from build123d import *

# Parameters (mm, degrees)
F1_DEPTH  = 12
F2_START  = 3
F2_DEPTH  = 6
F3_D      = 6.7564
F5_START  = -6
F5_DEPTH  = 4
F6_D      = 3.3
F6_DEPTH  = 8
F6_TIP    = 0.9914200214
F7_D      = 6
F7_DEPTH  = 1.5
F7_TIP    = 1.8025818571
F9_START  = -6
F9_DEPTH  = 4
F10_D     = 3.3
F10_DEPTH = 8
F10_TIP   = 0.9914200214
F11_D     = 6
F11_DEPTH = 1.5
F11_TIP   = 1.8025818571
F13_START = -6
F13_DEPTH = 4
F14_D     = 6
F14_DEPTH = 1.5
F14_TIP   = 1.8025818571
F15_D     = 3.3
F15_DEPTH = 8
F15_START = 2.3111618
F15_TIP   = 0.9914200214


with BuildPart() as f1:
    # F0 (on Front) → F1 (new body)
    with BuildSketch(Plane.XZ):
        with BuildLine():
            Line((3, -59.9289579419), (53.4, 27.3664027596))
            ThreePointArc((53.4, 27.3664027596), (51.2038475773, 29.5625551823), (50.4, 32.5625551823))
            Line((50.4, 32.5625551823), (-50.4, 32.5625551823))
            ThreePointArc((-50.4, 32.5625551823), (-51.2038475773, 29.5625551823), (-53.4, 27.3664027596))
            Line((-53.4, 27.3664027596), (-3, -59.9289579419))
            ThreePointArc((-3, -59.9289579419), (0, -59.1251103646), (3, -59.9289579419))
        make_face()
        Polygon((10, 24.5625551823), (42.5435935394, 24.5625551823), (26.2717967697, -3.6210235533), (16.2717967697, -20.941531629), (0, -49.1251103646), (-16.2717967697, -20.941531629), (-26.2717967697, -3.6210235533), (-42.5435935394, 24.5625551823), (-10, 24.5625551823), align=None, mode=Mode.SUBTRACT)
    extrude(amount=F1_DEPTH)



with BuildPart() as f1b:
    # F0 (on Front) → F1, piece 2 (new body)
    with BuildSketch(Plane.XZ):
        with BuildLine():
            ThreePointArc((5, -8.6602540378), (8.6602540378, -5), (10, 0))
            ThreePointArc((10, 0), (8.6602540378, 5), (5, 8.6602540378))
            ThreePointArc((5, 8.6602540378), (0, 10), (-5, 8.6602540378))
            ThreePointArc((-5, 8.6602540378), (-8.6602540378, 5), (-10, 0))
            ThreePointArc((-10, 0), (-8.6602540378, -5), (-5, -8.6602540378))
            ThreePointArc((-5, -8.6602540378), (0, -10), (5, -8.6602540378))
        make_face()
    extrude(amount=F1_DEPTH)


with BuildPart() as f1_1:
    add(f1.part)

    add(f1b.part)  # F2 merges F1b
    # F0 (on Front) → F2 (join)
    with BuildSketch(Plane.XZ.offset(F2_START)):
        with BuildLine():
            Line((10, 5.7735026919), (10, 24.5625551823))
            Line((10, 24.5625551823), (-10, 24.5625551823))
            Line((-10, 24.5625551823), (-10, 5.7735026919))
            Line((-10, 5.7735026919), (-5, 8.6602540378))
            ThreePointArc((-5, 8.6602540378), (0, 10), (5, 8.6602540378))
            Line((5, 8.6602540378), (10, 5.7735026919))
        make_face()
        with BuildLine():
            Line((16.2717967697, -20.941531629), (26.2717967697, -3.6210235533))
            Line((26.2717967697, -3.6210235533), (10, 5.7735026919))
            Line((10, 5.7735026919), (10, 0))
            ThreePointArc((10, 0), (8.6602540378, -5), (5, -8.6602540378))
            Line((5, -8.6602540378), (0, -11.5470053838))
            Line((0, -11.5470053838), (16.2717967697, -20.941531629))
        make_face()
        with BuildLine():
            Line((-16.2717967697, -20.941531629), (0, -11.5470053838))
            Line((0, -11.5470053838), (-5, -8.6602540378))
            ThreePointArc((-5, -8.6602540378), (-8.6602540378, -5), (-10, 0))
            Line((-10, 0), (-10, 5.7735026919))
            Line((-10, 5.7735026919), (-26.2717967697, -3.6210235533))
            Line((-26.2717967697, -3.6210235533), (-16.2717967697, -20.941531629))
        make_face()
        with BuildLine():
            Line((-5, 8.6602540378), (-10, 5.7735026919))
            Line((-10, 5.7735026919), (-10, 0))
            ThreePointArc((-10, 0), (-8.6602540378, 5), (-5, 8.6602540378))
        make_face()
        with BuildLine():
            Line((10, 0), (10, 5.7735026919))
            Line((10, 5.7735026919), (5, 8.6602540378))
            ThreePointArc((5, 8.6602540378), (8.6602540378, 5), (10, 0))
        make_face()
        with BuildLine():
            Line((-5, -8.6602540378), (0, -11.5470053838))
            Line((0, -11.5470053838), (5, -8.6602540378))
            ThreePointArc((5, -8.6602540378), (0, -10), (-5, -8.6602540378))
        make_face()
    extrude(amount=F2_DEPTH)

    # F3 (through all)
    with Locations(Plane(origin=(0, 0, 0), x_dir=(1, 0, 0), z_dir=(0, 1, 0))):
        with Locations((0, 0)):
            Hole(F3_D / 2)

    # F4 (on face) → F5 (cut)
    with BuildSketch(Plane(origin=(-28.2, 0, -16.2812775911), x_dir=(0, -1, 0), z_dir=(-0.8660254038, 0, -0.5)).offset(F5_START)):
        Polygon((8.9, -34.3256842194), (6, -32.6513684387), (3.1, -34.3256842194), (3.1, -37.6743157806), (6, -39.3486315613), (8.9, -37.6743157806), align=None)
        Polygon((3.1, -20.6743157806), (6, -22.3486315613), (8.9, -20.6743157806), (8.9, -17.3256842194), (6, -15.6513684387), (3.1, -17.3256842194), align=None)
        Polygon((8.9, 17.3256842194), (8.9, 20.6743157806), (6, 22.3486315613), (3.1, 20.6743157806), (3.1, 17.3256842194), (6, 15.6513684387), align=None)
        Polygon((6, 32.6513684387), (8.9, 34.3256842194), (8.9, 37.6743157806), (6, 39.3486315613), (3.1, 37.6743157806), (3.1, 34.3256842194), align=None)
    extrude(amount=-F5_DEPTH, mode=Mode.SUBTRACT)

    # F6
    with Locations(Plane(origin=(-28.2, 0, -16.2812775911), x_dir=(0, -1, 0), z_dir=(-0.8660254038, 0, -0.5))):
        with Locations((6, -36), (6, -19), (6, 19), (6, 36)):
            Hole(F6_D / 2, depth=F6_DEPTH)
            with Locations((0, 0, -(F6_DEPTH + F6_TIP / 2))):  # 118° drill point
                Cone(0, F6_D / 2, F6_TIP, mode=Mode.SUBTRACT)

    # F7
    with Locations(Plane(origin=(-28.2, 0, -16.2812775911), x_dir=(0, -1, 0), z_dir=(-0.8660254038, 0, -0.5))):
        with Locations((6, -36), (6, -19), (6, 19), (6, 36)):
            Hole(F7_D / 2, depth=F7_DEPTH)
            with Locations((0, 0, -(F7_DEPTH + F7_TIP / 2))):  # 118° drill point
                Cone(0, F7_D / 2, F7_TIP, mode=Mode.SUBTRACT)

    # F8 (on face) → F9 (cut)
    with BuildSketch(Plane.XY.offset(32.5625551823).offset(F9_START)):
        Polygon((-34.3256842194, -8.9), (-32.6513684387, -6), (-34.3256842194, -3.1), (-37.6743157806, -3.1), (-39.3486315613, -6), (-37.6743157806, -8.9), align=None)
        Polygon((-20.6743157806, -8.9), (-17.3256842194, -8.9), (-15.6513684387, -6), (-17.3256842194, -3.1), (-20.6743157806, -3.1), (-22.3486315613, -6), align=None)
        Polygon((34.3256842194, -8.9), (37.6743157806, -8.9), (39.3486315613, -6), (37.6743157806, -3.1), (34.3256842194, -3.1), (32.6513684387, -6), align=None)
        Polygon((20.943141643, -8.908812938), (22.6174574237, -6.008812938), (20.943141643, -3.108812938), (17.5945100817, -3.108812938), (15.9201943011, -6.008812938), (17.5945100817, -8.908812938), align=None)
    extrude(amount=-F9_DEPTH, mode=Mode.SUBTRACT)

    # F10
    with Locations(Plane.XY.offset(32.5625551823)):
        with Locations((-36, -6), (-19, -6), (19.2688258624, -6.008812938), (36, -6)):
            Hole(F10_D / 2, depth=F10_DEPTH)
            with Locations((0, 0, -(F10_DEPTH + F10_TIP / 2))):  # 118° drill point
                Cone(0, F10_D / 2, F10_TIP, mode=Mode.SUBTRACT)

    # F11
    with Locations(Plane.XY.offset(32.5625551823)):
        with Locations((-36, -6), (-19, -6), (19.2688258624, -6.008812938), (36, -6)):
            Hole(F11_D / 2, depth=F11_DEPTH)
            with Locations((0, 0, -(F11_DEPTH + F11_TIP / 2))):  # 118° drill point
                Cone(0, F11_D / 2, F11_TIP, mode=Mode.SUBTRACT)

    # F12 (on face) → F13 (cut)
    with BuildSketch(Plane(origin=(28.2, 0, -16.2812775911), x_dir=(0, 1, 0), z_dir=(0.8660254038, 0, -0.5)).offset(F13_START)):
        Polygon((-8.9, 34.3256842194), (-6, 32.6513684387), (-3.1, 34.3256842194), (-3.1, 37.6743157806), (-6, 39.3486315613), (-8.9, 37.6743157806), align=None)
        Polygon((-3.1, 20.6743157806), (-6, 22.3486315613), (-8.9, 20.6743157806), (-8.9, 17.3256842194), (-6, 15.6513684387), (-3.1, 17.3256842194), align=None)
        Polygon((-6, -15.6513684387), (-8.9, -17.3256842194), (-8.9, -20.6743157806), (-6, -22.3486315613), (-3.1, -20.6743157806), (-3.1, -17.3256842194), align=None)
        Polygon((-6, -32.6513684387), (-8.9, -34.3256842194), (-8.9, -37.6743157806), (-6, -39.3486315613), (-3.1, -37.6743157806), (-3.1, -34.3256842194), align=None)
    extrude(amount=-F13_DEPTH, mode=Mode.SUBTRACT)

    # F14
    with Locations(Plane(origin=(28.2, 0, -16.2812775911), x_dir=(0, 1, 0), z_dir=(0.8660254038, 0, -0.5))):
        with Locations((-6, 36), (-6, 19), (-6, -19), (-6, -36)):
            Hole(F14_D / 2, depth=F14_DEPTH)
            with Locations((0, 0, -(F14_DEPTH + F14_TIP / 2))):  # 118° drill point
                Cone(0, F14_D / 2, F14_TIP, mode=Mode.SUBTRACT)

    # F15
    # its depths count from where the whole tool has entered the part; down to there all is cleared
    with Locations(Plane(origin=(28.2, 0, -16.2812775911), x_dir=(0, 1, 0), z_dir=(0.8660254038, 0, -0.5)).offset(-F15_START)):
        with Locations((-6, 36), (-6, 19), (-6, -19), (-6, -36)):
            Hole(F15_D / 2, depth=F15_DEPTH)
            with Locations((0, 0, -(F15_DEPTH + F15_TIP / 2))):  # 118° drill point
                Cone(0, F15_D / 2, F15_TIP, mode=Mode.SUBTRACT)


solid = f1_1.part
Could you check a few things on this model? Use its own coordinates, in mm. A direction names the side the tool comes from. Give positions to 0.01 mm unless a question says otherwise; leave off trailing zeros. Return JSON: item names as keys, results as strings. Group by question number.
Q1. Which directions (+Z, -Z, +X, -X, +Y, -Y) give clear straight access to the entire face, cutting with the end or side of a thin tool? Please do faces 3 (the face through (-33, -6, 32)), 4 (the face through (38.888, -4.57, 16.203)), 5 (the face through (-12, -3, -3)).
Q2. Thinking about a two-plate mould opening in X: for faces 1 (the face through (2.681, -6.084, 2.056)), 2 (the face through (20, -12, -17)), which applies, pulls with the +X half, pulls with the -X half, needs draft (parallel to the pull), parting line crosses it, or undercut?
Q3. Please list where these lines run through material, in increasing order: line 1 along X through (y, z) = (-8.75, 10.5); line 2 along X through (y, z) = (-6, 27.4); line 3 along Z through (x, y) = (3, -3.75). Write a range as [from, to].
Q4. Will these pins go through, and if not, where does the flat tip stop? pin 1 Ø6.5 at (y, z) = (-5, 14) entering from +X; pin 2 Ø2 at (y, z) = (-2.5, -47) entering from +X; pin 3 Ø1.5 at (x, y) = (4, -1.5) entering from -Z; pin 4 Ø4 at (x, z) = (0, 0) entering from +Y.
Resolved:
{
 "1": {"face 3": "+Z", "face 4": "none", "face 5": "+Y"},
 "2": {"face 1": "undercut", "face 2": "needs draft"},
 "3": {"line 1": "x = [-43.66, -34.42], [-10, 10], [34.42, 43.66]", "line 2": "x = [-53.34, -37.65], [-34.35, -20.65], [-17.35, 17.62], [20.92, 34.35], [37.65, 53.34]", "line 3": "z = [-59.93, -45.67], [-13.28, -1.55], [1.55, 32.56]"},
 "4": {"pin 1": "stops at x = 47.55", "pin 2": "stops at x = 11.04", "pin 3": "stops at z = -59.5", "pin 4": "passes through"}
}
